from build123d import *

# Parameters (mm, degrees)
CROQUIS1_R                 = 5
SALIENTE_EXTRUIR1_DEPTH    = 10
SALIENTE_EXTRUIR2_START    = 6.6
CROQUIS3_R                 = 1.5
SALIENTE_EXTRUIR2_DEPTH    = 2
SALIENTE_EXTRUIR3_START    = -3.3
CROQUIS3_3_R               = 1.5
SALIENTE_EXTRUIR3_DEPTH    = 2.9
SALIENTE_EXTRUIR4_START    = -1.1
SALIENTE_EXTRUIR4_DEPTH    = 5.1
SALIENTE_EXTRUIR5_START    = -6.2
SALIENTE_EXTRUIR5_DEPTH    = 14.8
CORTAR_EXTRUIR1_DEPTH      = 31
SALIENTE_EXTRUIR6_DEPTH    = 10
CROQUIS5_R                 = 1.5
CORTAR_EXTRUIR2_DEPTH      = 15.8
CHAFL_N1_SIZE              = 1.45
CHAFL_N1_SIZE2             = 1.8
CHAFL_N2_SIZE              = 1.45
CHAFL_N2_SIZE2             = 1.8
REDONDEO1_R                = 4
CORTAR_EXTRUIR3_DEPTH      = 8.159143338
CORTAR_EXTRUIR3_DEPTH_BACK = 8.159143338


with BuildPart() as part:
    # Croquis1 → Saliente-Extruir1 (new body)
    with BuildSketch(Plane(origin=(0, 0, 0), x_dir=(1, 0, 0), z_dir=(0, 1, 0))):
        Polygon((7.159143338, 0), (3.579571669, 6.2), (-3.579571669, 6.2), (-7.159143338, 0), (-3.579571669, -6.2), (3.579571669, -6.2), align=None)
        Circle(CROQUIS1_R, mode=Mode.SUBTRACT)
    extrude(amount=-SALIENTE_EXTRUIR1_DEPTH)



with BuildPart() as body_2:
    # Croquis3 → Saliente-Extruir2 (new body)
    with BuildSketch(Plane.XY.offset(SALIENTE_EXTRUIR2_START)):
        with BuildLine():
            Line((-4, 6), (-4, 20))
            Line((-4, 20), (4, 20))
            Line((4, 20), (4, 6))
            ThreePointArc((4, 6), (0, 2), (-4, 6))
        make_face()
        with BuildLine():
            ThreePointArc((3.2, 10), (0, 13.2), (-3.2, 10))
            Line((-3.2, 10), (-3.2, 6))
            ThreePointArc((-3.2, 6), (0, 2.8), (3.2, 6))
            Line((3.2, 6), (3.2, 10))
        make_face(mode=Mode.SUBTRACT)
        with BuildLine():
            Line((3.2, 6), (3.2, 10))
            ThreePointArc((3.2, 10), (0, 13.2), (-3.2, 10))
            Line((-3.2, 10), (-3.2, 6))
            ThreePointArc((-3.2, 6), (0, 2.8), (3.2, 6))
        make_face()
        with Locations((0, 6)):
            Circle(CROQUIS3_R, mode=Mode.SUBTRACT)
        with Locations((0, 10)):
            Circle(CROQUIS3_R, mode=Mode.SUBTRACT)
        with Locations((0, 6)):
            Circle(CROQUIS3_R)
    extrude(amount=SALIENTE_EXTRUIR2_DEPTH)


with BuildPart() as body_3:
    # Croquis3<3> → Saliente-Extruir3 (new body)
    with BuildSketch(Plane.XY.offset(SALIENTE_EXTRUIR3_START)):
        with BuildLine():
            Line((3.2, 6), (3.2, 10))
            ThreePointArc((3.2, 10), (0, 13.2), (-3.2, 10))
            Line((-3.2, 10), (-3.2, 6))
            ThreePointArc((-3.2, 6), (0, 2.8), (3.2, 6))
        make_face()
        with Locations((0, 6)):
            Circle(CROQUIS3_3_R, mode=Mode.SUBTRACT)
        with Locations((0, 10)):
            Circle(CROQUIS3_3_R, mode=Mode.SUBTRACT)
        with Locations((0, 10)):
            Circle(CROQUIS3_3_R)
    extrude(amount=-SALIENTE_EXTRUIR3_DEPTH)

    # Croquis3<4> → Saliente-Extruir4 (add)
    with BuildSketch(Plane.XY.offset(SALIENTE_EXTRUIR4_START)):
        with BuildLine():
            Line((-4, 6), (-4, 20))
            Line((-4, 20), (4, 20))
            Line((4, 20), (4, 6))
            ThreePointArc((4, 6), (0, 2), (-4, 6))
        make_face()
        with BuildLine():
            ThreePointArc((3.2, 10), (0, 13.2), (-3.2, 10))
            Line((-3.2, 10), (-3.2, 6))
            ThreePointArc((-3.2, 6), (0, 2.8), (3.2, 6))
            Line((3.2, 6), (3.2, 10))
        make_face(mode=Mode.SUBTRACT)
    extrude(amount=-SALIENTE_EXTRUIR4_DEPTH)


with BuildPart() as part_1:
    add(part.part)

    add(body_2.part)  # Saliente-Extruir5 merges body 2

    add(body_3.part)  # Saliente-Extruir5 merges body 3
    # Croquis3<6> → Saliente-Extruir5 (add)
    with BuildSketch(Plane.XY.offset(SALIENTE_EXTRUIR5_START)):
        with BuildLine():
            ThreePointArc((-4, 6), (0, 2), (4, 6))
            Line((4, 6), (4, 20))
            Line((4, 20), (7.159143338, 20))
            Line((7.159143338, 20), (7.159143338, 0))
            Line((7.159143338, 0), (-7.159143338, 0))
            Line((-7.159143338, 0), (-7.159143338, 20))
            Line((-7.159143338, 20), (-4, 20))
            Line((-4, 20), (-4, 6))
        make_face()
    extrude(amount=SALIENTE_EXTRUIR5_DEPTH)

    # Croquis4 → Cortar-Extruir1 (cut, through all)
    with BuildSketch(Plane(origin=(0, -10, 0), x_dir=(-1, 0, 0), z_dir=(0, -1, 0))):
        Polygon((7.159143338, 6.2), (7.159143338, 0), (3.579571669, 6.2), align=None)
        Polygon((-7.159143338, 6.2), (-3.579571669, 6.2), (-7.159143338, 0), align=None)
    extrude(amount=-CORTAR_EXTRUIR1_DEPTH, mode=Mode.SUBTRACT)

    # Croquis4<3> → Saliente-Extruir6 (add)
    with BuildSketch(Plane(origin=(0, -10, 0), x_dir=(-1, 0, 0), z_dir=(0, -1, 0))):
        Polygon((-7.159143338, -8.6), (7.159143338, -8.6), (7.159143338, 0), (3.579571669, -6.2), (-3.579571669, -6.2), (-7.159143338, 0), align=None)
    extrude(amount=-SALIENTE_EXTRUIR6_DEPTH)

    # Croquis5 → Cortar-Extruir2 (cut, through all)
    with BuildSketch(Plane(origin=(0, 0, -6.2), x_dir=(-1, 0, 0), z_dir=(0, 0, -1))):
        with Locations((0, -5)):
            Circle(CROQUIS5_R)
    extrude(amount=-CORTAR_EXTRUIR2_DEPTH, mode=Mode.SUBTRACT)

    # Chaflán1
    chafl_n1_edges = [part_1.edges().sort_by_distance(p)[0] for p in [
        (-1.5, 10, 8.6),
    ]]
    chafl_n1_side = [part_1.faces().sort_by_distance(p)[0] for p in [
        (0, 5.085079308, 8.6),
    ]]
    chamfer(chafl_n1_edges, length=CHAFL_N1_SIZE, length2=CHAFL_N1_SIZE2, reference=chafl_n1_side[0])

    # Chaflán2
    chafl_n2_edges = [part_1.edges().sort_by_distance(p)[0] for p in [
        (-1.5, 6, -6.2),
    ]]
    chafl_n2_side = [part_1.faces().sort_by_distance(p)[0] for p in [
        (-1.5, 6, -4.75),
    ]]
    chamfer(chafl_n2_edges, length=CHAFL_N2_SIZE, length2=CHAFL_N2_SIZE2, reference=chafl_n2_side[0])

    # Redondeo1
    redondeo1_edges = [part_1.edges().sort_by_distance(p)[0] for p in [
        (7.159143338, 5, 8.6),
        (-7.159143338, 5, 8.6),
    ]]
    fillet(redondeo1_edges, radius=REDONDEO1_R)

    # Croquis6 → Cortar-Extruir3 (cut, two sides)
    with BuildSketch(Plane(origin=(0, 0, 0), x_dir=(0, 0, -1), z_dir=(1, 0, 0))) as cortar_extruir3_sk:
        Polygon((6.2, 20), (0.2, 20), (6.2, 11), align=None)
    extrude(amount=CORTAR_EXTRUIR3_DEPTH, mode=Mode.SUBTRACT)
    extrude(cortar_extruir3_sk.sketch, amount=-CORTAR_EXTRUIR3_DEPTH_BACK, mode=Mode.SUBTRACT)


solid = part_1.part
The listing builds one solid part. Answer for the finished solid, in the listing's coordinates (mm). A direction names the side the tool comes from. Give positions to 0.01 mm unless a question says otherwise; leave off trailing zeros. Write each loop counter-clockwise with the first axis right and the second up, starting at its lowest first coordinate (ties: lowest second). Pieces come first, ordered by that corner, then holes. Notation, with made-up numbers: (87, -40) -> (143, -40) arc R21 cw to (143, -32) -> close; hole circle Ø9 at (-31, -25.5). An arc over 180 degrees is marked (long way). One line per question, with ' | ' between items. Start each with the question number.
1. Find the intervals of material crossed by probe 1 along Y at (x, z) = (0, 7.2); probe 2 along Y at (x, z) = (0, 7.6); probe 3 along Z at (x, y) = (0, -8), in increasing order.
2. Section A-A (y = -7) is taken. Determine the outline of the cut face in (x, z).
3. Section D-D (z = 2) is taken. Determine the outline of the cut face in (x, y), plus the area to 3 significant figures.
4. Section C-C (x = 0) is taken. State how many separate pieces and enclosed holes the cut face has, plus the area to 3 significant figures.
5. Given pin 1 Ø1 at (y, z) = (10.5, -1) entering from -X; pin 2 Ø4 at (x, y) = (5.5, 12) entering from -Z; pin 3 Ø1.8 at (y, z) = (9, -1.5) entering from +X; pin 4 Ø1.8 at (x, y) = (0, -5) entering from -Z, each flat-ended and moving along its own axis, determine where each tip first touches the part or whether it passes through.
6. Section B-B (y = 1) is taken. Determine the outline of the cut face in (x, z), plus the area to 3 significant figures.
7. For faces 1 (the flat face through (4, 13, 3)), 2 (the cylindrical face through (-0.1, 2.8, -2.2)), 3 (the flat face through (0, 0, 0)), determine the directions among +Z, -Z, +X, -X, +Y, -Y from which every point of the face is accessible in a straight line to the end or side of a thin tool.
8. For a pull along X with two mould halves and no side action, classify faces 4 (the cylindrical face through (5.956, 5.21, 7.459)), 5 (the flat face through (0, -10, 6)), 6 (the flat face through (-7.159, 5, 2)), 7 (the cylindrical face through (0.1, 13.2, -2.2)) as pulls with the +X half, pulls with the -X half, needs draft (parallel to the pull), parting line crosses it, or undercut.
Response values:
1) probe 1: -10 to -6.5, -3.5 to 8.18, 11.82 to 20 | probe 2: -10 to -6.5, -3.5 to 7.86, 12.14 to 20 | probe 3: -6.2 to -5, 5 to 8.6
2) outline: (-7.16, 0) -> (-3.58, -6.2) -> (3.58, -6.2) -> (7.16, 0) -> (7.16, 4.6) arc R4 ccw to (3.16, 8.6) -> (-3.16, 8.6) arc R4 ccw to (-7.16, 4.6) -> close; hole circle Ø10 at (0, 0)
3) outline: (-7.16, -10) -> (-4.58, -10) -> (-4.58, 0) -> (4.58, 0) -> (4.58, -10) -> (7.16, -10) -> (7.16, 20) -> (4, 20) -> (4, 6) arc R4 cw to (-4, 6) -> (-4, 20) -> (-7.16, 20) -> close | area: 201 mm2
4) separate pieces: 5 | enclosed holes: 0 | area: 122 mm2
5) pin 1: x = -6.87 | pin 2: z = -6.06 | pin 3: x = 6.81 | pin 4: through
6) outline: (-7.16, 0) -> (-3.58, -6.2) -> (3.58, -6.2) -> (7.16, 0) -> (7.16, 4.6) arc R4 ccw to (3.16, 8.6) -> (-3.16, 8.6) arc R4 ccw to (-7.16, 4.6) -> close | area: 183 mm2
7) face 1: +Y | face 2: none | face 3: -Y
8) face 4: pulls with the +X half | face 5: needs draft | face 6: pulls with the -X half | face 7: undercut
